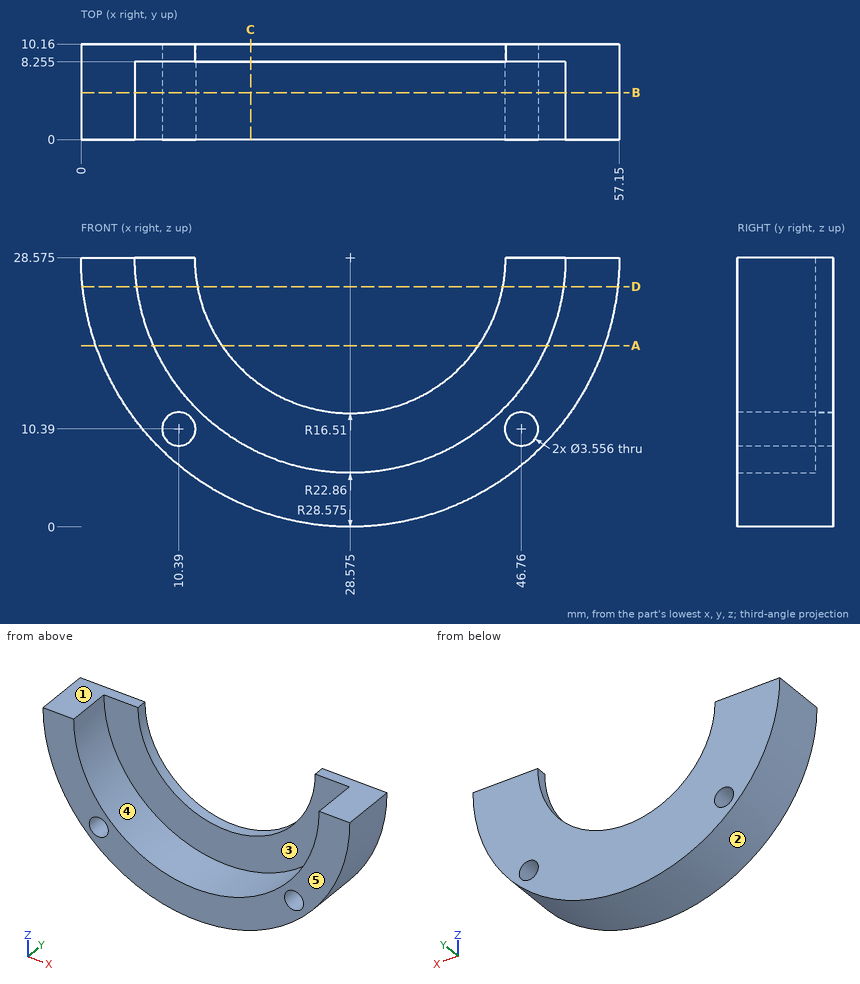
Print and shaded views of the part. All mm, measured from the part's lowest x, y and z. A direction names the side the tool comes from. Give positions to 0.01 mm unless a question says otherwise; leave off trailing zeros. Order: outer loops, then holes, each group sorted by start corner. A loop starts at its lowest first (then second) coordinate and runs counter-clockwise, first axis right, second up. Notation, with made-up numbers: M -40,-28.75 L 0,-28.75 A20 ccw 0,-18.75 Z; hole C 21,41 d8. An arc over 180 degrees is marked long. Use one line per item in the form item = value.
Q1. Slice it at D-D, the plane z = 25.5. Write the cut outline in (x, y) (3 decimals), and give its area (3 significant figures).
Conclusion:
outline = M 0.166,0 L 5.923,0 L 5.923,8.255 L 12.354,8.255 L 12.354,10.16 L 0.166,10.16 Z; M 44.796,8.255 L 51.227,8.255 L 51.227,0 L 56.984,0 L 56.984,10.16 L 44.796,10.16 Z
area = 141 mm2
Q2. Pull direction X, two halves, no side cores. Call the marked faces 1, 2 and 3: released by +X, released by -X, zero draft, split by the parting line, or undercut.
Conclusion:
face_1 = zero draft
face_2 = split by the parting line
face_3 = undercut
Q3. Pin check, flat tips, straight feed: P1, Ø6, axis at y = 7.5, z = 8, coming from the +X side; P2, Ø7, axis at x = 35.5, z = 16.5, coming from the -Y side (3 decimals); P3, Ø4, axis at x = 33.5, y = 1.5, coming from the +Z side. Stop position of each tip, or through.
Conclusion:
P1 = 51.11
P2 = 8.255
P3 = 6.79
Q4. Which spindle directions (+Z, -Z, +X, -X, +Y, -Y) get a long thin tool onto all of the face, cutting with end or side? Do the marked faces 4 and 5. Say none if no direction does.
Conclusion:
face_4 = +Z, -Y
face_5 = +Z, -Z, +X, -X, -Y
Q5. Slice it at C-C, the plane x = 18. Write the cut outline in (y, z) (3 decimals), and give its area (3 significant figures).
Conclusion:
outline = M 0,2.029 L 10.16,2.029 L 10.16,15.896 L 8.255,15.896 L 8.255,8.308 L 0,8.308 Z
area = 78.3 mm2
Q6. Slice it at B-B, the plane y = 5. Write the cut outline in (x, z) (3 decimals).
Conclusion:
outline = M 0,28.575 A28.575 ccw 57.15,28.575 L 51.435,28.575 A22.86 cw 5.715,28.575 Z; hole C 10.39,10.39 d3.556; hole C 46.76,10.39 d3.556
Q7. Slice it at A-A, the plane z = 19.25. Write the cut outline in (x, y) (3 decimals).
Conclusion:
outline = M 1.564,0 L 7.703,0 L 7.703,8.255 L 14.951,8.255 L 14.951,10.16 L 1.564,10.16 Z; M 42.199,8.255 L 49.447,8.255 L 49.447,0 L 55.586,0 L 55.586,10.16 L 42.199,10.16 Z
Q8. Wall check: probe 1 along X at (y, z) = (6.5, 11); probe 2 along Y at (x, z) = (14, 20.5) (3 decimals); probe 3 along X at (y, z) = (2.75, 16.5). Give the ranges that are in metal, low to high.
Conclusion:
probe_1 = 6.04 to 8.72, 12.06 to 13.96, 43.19 to 45.09, 48.43 to 51.11
probe_2 = 8.255 to 10.16
probe_3 = 2.68 to 9.16, 47.99 to 54.47
